Autodesk Inventor part; units mm, degrees
ref_plane "YZ Plane" through (0, 0, 0) normal (1, 0, 0) x (0, 1, 0)
ref_plane "XZ Plane" through (0, 0, 0) normal (0, 1, 0) x (-1, 0, 0)
ref_plane "XY Plane" through (0, 0, 0) normal (0, 0, 1) x (1, 0, 0)
sketch "Sketch1" plane through (0, 0, 0) normal (0, 0, 1) x (1, 0, 0)
  line L0 (0, 0) -> (10, 0)
  line L1 (10, 0) -> (10, 10)
  line L2 (10, 10) -> (0, 10)
  line L3 (0, 10) -> (0, 0)
  dimension "d0" = 10
  dimension "d1" = 10
extrude "Extrusion1" add sketch "Sketch1" along normal blind 4.5
sketch "Sketch2" plane through (0, 0, 0) normal (0, -1, 0) x (1, 0, 0)
  line L0 (0, 0) -> (0, 4.5)
  line L1 (0, 0) -> (10, 0)
  line L2 (10, 0) -> (10, 4.5)
  line L3 (1.8, 0) -> (1.8, 3.6067)
  line L4 (2.8, 0) -> (1.9843, 3.6272)
  line L5 (7.2, 0) -> (8.0157, 3.6272)
  line L6 (8.2, 3.6067) -> (8.2, 0)
  arc A0 (1.9843, 3.6272) -> (1.8, 3.6067) centre (1.8933, 3.6067) ccw
  arc A1 (8.2, 3.6067) -> (8.0157, 3.6272) centre (8.1067, 3.6067) ccw
  line L7 (0, 3.7) -> (10, 3.7) construction
  line L8 (3.862, 3.7) -> (6.138, 3.7)
  line L9 (6.138, 3.7) -> (6.138, 1)
  line L10 (6.138, 1) -> (3.862, 1)
  line L11 (3.862, 1) -> (3.862, 3.7)
  dimension "d9" = 1
  dimension "d10" = 1
  dimension "d11" = 3.7
  dimension "d12" = 4.4
  dimension "d13" = 1.8
  dimension "d14" = 1.8
  dimension "d15" = 3.862
  dimension "d16" = 3.862
  dimension "d17" = 1
extrude "Extrusion2" cut sketch "Sketch2" against normal through all
sketch "Sketch3" plane through (0, 0, 0) normal (-1, 0, 0) x (0, 0, 1)
  line L0 (0, 10) -> (4.5, 10)
  line L1 (0, 10) -> (0, 0)
  line L2 (0, 0) -> (4.5, 0)
  line L3 (0, 10) -> (4.2679, 10)
  line L4 (0, 10) -> (0, 0)
  line L5 (0, 0) -> (4.0987, 0)
  line L6 (0, 8.2) -> (3.4545, 8.2)
  line L7 (0, 7.2) -> (3.4901, 7.7116)
  line L8 (0, 2.8) -> (3.4901, 2.2884)
  line L9 (3.4545, 1.8) -> (0, 1.8)
  arc A0 (3.4901, 7.7116) -> (3.4545, 8.2) centre (3.4545, 7.9545) ccw
  arc A1 (3.4545, 1.8) -> (3.4901, 2.2884) centre (3.4545, 2.0455) ccw
  line L10 (3.7, 10) -> (3.7, 0) construction
  line L11 (3.7, 6.138) -> (3.7, 3.862)
  line L12 (3.7, 3.862) -> (1, 3.862)
  line L13 (1, 3.862) -> (1, 6.138)
  line L14 (1, 6.138) -> (3.7, 6.138)
  dimension "d20" = 1
  dimension "d21" = 1
  dimension "d22" = 3.7
  dimension "d23" = 4.4
  dimension "d24" = 1.8
  dimension "d25" = 1.8
  dimension "d26" = 3.862
  dimension "d27" = 3.862
  dimension "d28" = 1
extrude "Extrusion3" cut sketch "Sketch3" against normal through all
sketch "Sketch4" plane through (0, 0, 0) normal (0, 0, -1) x (-1, 0, 0)
  line L0 (-2.8, 7.2) -> (-7.2, 7.2)
  line L1 (-7.2, 7.2) -> (-7.2, 2.8)
  line L2 (-7.2, 2.8) -> (-2.8, 2.8)
  line L3 (-2.8, 2.8) -> (-2.8, 7.2)
  line L4 (-0.5, 9.5) -> (-9.5, 9.5)
  line L5 (-9.5, 9.5) -> (-9.5, 0.5)
  line L6 (-9.5, 0.5) -> (-0.5, 0.5)
  line L7 (-0.5, 0.5) -> (-0.5, 9.5)
  line L8 (-2.8, 7.2) -> (-7.2, 2.8) construction
  line L9 (-5, 7.2) -> (-5, 2.8) construction
  line L10 (-2.8, 5) -> (-7.2, 5) construction
  point P0 (0, 0)
  dimension "d32" = 4.5
  dimension "d33" = 4.5
  dimension "d34" = 4.5
extrude "Extrusion4" cut sketch "Sketch4" against normal blind 4 contours L3 L2 L1 L0 | L7 L6 L5 L4
sketch "Sketch5" plane through (0, 0, 4.5) normal (0, 0, 1) x (1, 0, 0)
  line L0 (0, 0) -> (0, 10)
  line L1 (0, 10) -> (10, 10)
  circle A0 centre (5, 5) radius 4
  dimension "d37" = 5
  dimension "d38" = 5
  dimension "d39" = 8
extrude "Extrusion5" add sketch "Sketch5" along normal blind 3.5
fillet "Fillet1" radius 0.5 1 edges at (1, 5, 8)
chamfer "Chamfer1" distance 0.2 angle 45 4 edges at (5, 10, 4.5) (0, 5, 4.5) (10, 5, 4.5) (5, 0, 4.5)
equation "\"d13\" = d14"
equation "\"d15\" = d16"
equation "\"d24\" = d25"
equation "\"d26\" = d27"
equation "\"d33\" = d32"
equation "\"d34\" = d32"
properties part number "button_cap"
Design review of the part built by this model. Coordinates are the model's own, in mm. A direction names the side the tool comes from. Coordinates: 2 decimals unless noted, no trailing zeros. Loops run counter-clockwise (first coordinate to the right, second up) from the corner with the lowest first, then second, coordinate; pieces in that order, holes last. Notation, with made-up numbers: (70, 11) -> (79, 11) arc R17 cw to (79, 28) -> close; hole circle Ø1 at (46.25, 16.5). An arc over 180 degrees is marked (long way). Answer as a JSON object with one key per item and string values.
Q1. Take a section at A-A on y = 5. Give the boundary of the cut face in (x, z), plus the area to 3 significant figures.
Answer block:
{"outline": "(0, 0) -> (0.5, 0) -> (0.5, 1) -> (0, 1) -> close; (0, 3.7) -> (0.5, 3.7) -> (0.5, 4) -> (9.5, 4) -> (9.5, 3.7) -> (10, 3.7) -> (10, 4.3) -> (9.8, 4.5) -> (9, 4.5) -> (9, 7.5) arc R0.5 ccw to (8.5, 8) -> (1.5, 8) arc R0.5 ccw to (1, 7.5) -> (1, 4.5) -> (0.2, 4.5) -> (0, 4.3) -> close; (9.5, 0) -> (10, 0) -> (10, 1) -> (9.5, 1) -> close", "area": "34.2 mm^2"}
Q2. Tool access review of faces 4 (the flat face through (7.602, 9.746, 1.788)), 5 (the flat face through (0.7, 5.1, 4.5)), 6 (the flat face through (5, 5, 8)), 7 (the flat face through (0.3, 0.7, 0)), 8 (the flat face through (5, 5, 4)): name each direction out of +Z, -Z, +X, -X, +Y, -Y from which nothing blocks a thin tool from reaching the whole face with its end or side.
Answer block:
{"face 4": "-Z, +Y, -Y", "face 5": "+Z", "face 6": "+Z, +X, -X, +Y, -Y", "face 7": "-Z, +X, -X, +Y, -Y", "face 8": "-Z"}
Q3. The part is to be moulded in two halves that separate along Y. For faces 1 (the cylindrical face through (4.133, 8.905, 5.979)), 2 (the flat face through (0.5, 4.9, 0.6)), 3 (the flat face through (0, 5.1, 0.7)), say which applies: +Y half, -Y half, draft (parallel to the pull), parting line (faces both ways), or undercut.
Answer block:
{"face 1": "parting line", "face 2": "undercut", "face 3": "draft"}
Q4. Take a section at D-D on z = 6.75. Give the boundary of the cut face in (x, y), plus the area to 3 significant figures.
Answer block:
{"outline": "circle Ø8 at (5, 5)", "area": "50.3 mm^2"}
Q5. Take a section at C-C on z = 1.75. Give the number of separate pieces and of enclosed holes in the cut face, plus the area to 3 significant figures.
Answer block:
{"separate pieces": "12", "enclosed holes": "0", "area": "11.7 mm^2"}
Q6. To check wall thickness, follow L1, parallel to X at y = 6.5, z = 1.75; L2, parallel to Z at x = 1.75, y = 4.75; L3, parallel to Z at x = 4.25, y = 9. State the ranges of each line that lie inside material, in increasing order.
Answer block:
{"L1": "x = 0 to 0.5, 9.5 to 10", "L2": "z = 4 to 8", "L3": "z = 4 to 4.5"}
